```python
from build123d import *

# Parameters (mm, degrees)
SKETCH1_W             = 30
SKETCH1_H             = 18
BOSS_EXTRUDE1_DEPTH   = 30
SKETCH2_R             = 1.25
CUT_EXTRUDE1_DEPTH    = 8
SKETCH3_R             = 4
CUT_EXTRUDE2_DEPTH    = 6.5
SKETCH4_R             = 2.1
CUT_EXTRUDE3_DEPTH    = 24.5
CUT_EXTRUDE4_REACH    = 32
SKETCH5_W             = 12
SKETCH5_H             = 2.5
SKETCH6_R             = 3.45
CUT_EXTRUDE5_DEPTH    = 14
SKETCH7_R             = 1.25
CUT_EXTRUDE6_DEPTH    = 19
CHAMFER1_SIZE         = 1.7
CHAMFER1_SIZE2        = 0.65256886
CHAMFER1_PART_2_SIZE  = 1.7
CHAMFER1_PART_2_SIZE2 = 0.65256886


with BuildPart() as part:
    # Sketch1 → Boss-Extrude1 (new body)
    with BuildSketch(Plane(origin=(0, 0, 0), x_dir=(1, 0, 0), z_dir=(0, 1, 0))):
        Rectangle(SKETCH1_W, SKETCH1_H)
    extrude(amount=BOSS_EXTRUDE1_DEPTH)

    # Sketch2 → Cut-Extrude1 (cut)
    with BuildSketch(Plane(origin=(0, 30, 0), x_dir=(1, 0, 0), z_dir=(0, 1, 0))):
        with Locations((0, -6)):
            Circle(SKETCH2_R)
        with Locations((-8.5, 6)):
            Circle(SKETCH2_R)
        with Locations((8.5, 6)):
            Circle(SKETCH2_R)
    extrude(amount=-CUT_EXTRUDE1_DEPTH, mode=Mode.SUBTRACT)

    # Sketch3 → Cut-Extrude2 (cut)
    with BuildSketch(Plane(origin=(0, 30, 0), x_dir=(1, 0, 0), z_dir=(0, 1, 0))):
        with Locations((-9, -3)):
            Circle(SKETCH3_R)
        with Locations((9, -3)):
            Circle(SKETCH3_R)
    extrude(amount=-CUT_EXTRUDE2_DEPTH, mode=Mode.SUBTRACT)

    # Sketch4 → Cut-Extrude3 (cut, through all)
    with BuildSketch(Plane(origin=(0, 23.5, 0), x_dir=(1, 0, 0), z_dir=(0, 1, 0))):
        with Locations((9, -3)):
            Circle(SKETCH4_R)
        with Locations((-9, -3)):
            Circle(SKETCH4_R)
    extrude(amount=-CUT_EXTRUDE3_DEPTH, mode=Mode.SUBTRACT)

    # Sketch5 → Cut-Extrude4 (cut, up to next)
    with BuildSketch(Plane(origin=(15, 0, 0), x_dir=(0, 0, -1), z_dir=(1, 0, 0)), mode=Mode.PRIVATE) as cut_extrude4_sk1:
        with Locations((9, 7)):
            Rectangle(SKETCH5_W, SKETCH5_H)
    cut_extrude4_tool1 = extrude(cut_extrude4_sk1.sketch, amount=-CUT_EXTRUDE4_REACH, mode=Mode.PRIVATE) & part.part
    add(cut_extrude4_tool1.solids().sort_by_distance((15, 7, -9))[0], mode=Mode.SUBTRACT)
    # Sketch5 → Cut-Extrude4 (cut, up to next)
    with BuildSketch(Plane(origin=(15, 0, 0), x_dir=(0, 0, -1), z_dir=(1, 0, 0)), mode=Mode.PRIVATE) as cut_extrude4_sk2:
        with Locations((9, 11)):
            Rectangle(SKETCH5_W, SKETCH5_H)
    cut_extrude4_tool2 = extrude(cut_extrude4_sk2.sketch, amount=-CUT_EXTRUDE4_REACH, mode=Mode.PRIVATE) & part.part
    add(cut_extrude4_tool2.solids().sort_by_distance((15, 11, -9))[0], mode=Mode.SUBTRACT)
    # Sketch5 → Cut-Extrude4 (cut, up to next)
    with BuildSketch(Plane(origin=(15, 0, 0), x_dir=(0, 0, -1), z_dir=(1, 0, 0)), mode=Mode.PRIVATE) as cut_extrude4_sk3:
        with Locations((9, 15)):
            Rectangle(SKETCH5_W, SKETCH5_H)
    cut_extrude4_tool3 = extrude(cut_extrude4_sk3.sketch, amount=-CUT_EXTRUDE4_REACH, mode=Mode.PRIVATE) & part.part
    add(cut_extrude4_tool3.solids().sort_by_distance((15, 15, -9))[0], mode=Mode.SUBTRACT)
    # Sketch5 → Cut-Extrude4 (cut, up to next)
    with BuildSketch(Plane(origin=(15, 0, 0), x_dir=(0, 0, -1), z_dir=(1, 0, 0)), mode=Mode.PRIVATE) as cut_extrude4_sk4:
        with Locations((9, 19)):
            Rectangle(SKETCH5_W, SKETCH5_H)
    cut_extrude4_tool4 = extrude(cut_extrude4_sk4.sketch, amount=-CUT_EXTRUDE4_REACH, mode=Mode.PRIVATE) & part.part
    add(cut_extrude4_tool4.solids().sort_by_distance((15, 19, -9))[0], mode=Mode.SUBTRACT)
    # Sketch5 → Cut-Extrude4 (cut, up to next)
    with BuildSketch(Plane(origin=(15, 0, 0), x_dir=(0, 0, -1), z_dir=(1, 0, 0)), mode=Mode.PRIVATE) as cut_extrude4_sk5:
        with Locations((9, 23)):
            Rectangle(SKETCH5_W, SKETCH5_H)
    cut_extrude4_tool5 = extrude(cut_extrude4_sk5.sketch, amount=-CUT_EXTRUDE4_REACH, mode=Mode.PRIVATE) & part.part
    add(cut_extrude4_tool5.solids().sort_by_distance((15, 23, -9))[0], mode=Mode.SUBTRACT)
    # Sketch5 → Cut-Extrude4 (cut, up to next)
    with BuildSketch(Plane(origin=(15, 0, 0), x_dir=(0, 0, -1), z_dir=(1, 0, 0)), mode=Mode.PRIVATE) as cut_extrude4_sk6:
        with Locations((9, 27)):
            Rectangle(SKETCH5_W, SKETCH5_H)
    cut_extrude4_tool6 = extrude(cut_extrude4_sk6.sketch, amount=-CUT_EXTRUDE4_REACH, mode=Mode.PRIVATE) & part.part
    add(cut_extrude4_tool6.solids().sort_by_distance((15, 27, -9))[0], mode=Mode.SUBTRACT)
    # Sketch5 → Cut-Extrude4 (cut, up to next)
    with BuildSketch(Plane(origin=(15, 0, 0), x_dir=(0, 0, -1), z_dir=(1, 0, 0)), mode=Mode.PRIVATE) as cut_extrude4_sk7:
        with Locations((9, 3)):
            Rectangle(SKETCH5_W, SKETCH5_H)
    cut_extrude4_tool7 = extrude(cut_extrude4_sk7.sketch, amount=-CUT_EXTRUDE4_REACH, mode=Mode.PRIVATE) & part.part
    add(cut_extrude4_tool7.solids().sort_by_distance((15, 3, -9))[0], mode=Mode.SUBTRACT)

    # Sketch6 → Cut-Extrude5 (cut)
    with BuildSketch(Plane.XZ):
        with Locations((9, 3)):
            Circle(SKETCH6_R)
        with Locations((-9, 3)):
            Circle(SKETCH6_R)
    extrude(amount=-CUT_EXTRUDE5_DEPTH, mode=Mode.SUBTRACT)

    # Sketch7 → Cut-Extrude6 (cut, through all)
    with BuildSketch(Plane.XY.offset(9)):
        with Locations((-4.5, 20)):
            Circle(SKETCH7_R)
        with Locations((4.5, 20)):
            Circle(SKETCH7_R)
        with Locations((-9, 11)):
            Circle(SKETCH7_R)
        with Locations((-9, 3)):
            Circle(SKETCH7_R)
        with Locations((9, 11)):
            Circle(SKETCH7_R)
        with Locations((9, 3)):
            Circle(SKETCH7_R)
        with Locations((0, 10)):
            Circle(SKETCH7_R)
    extrude(amount=-CUT_EXTRUDE6_DEPTH, mode=Mode.SUBTRACT)

    # Chamfer1
    chamfer1_edges = [part.edges().sort_by_distance(p)[0] for p in [
        (6.9, 23.5, 3),
    ]]
    chamfer1_side = [part.faces().sort_by_distance(p)[0] for p in [
        (5.113137085, 23.5, 3),
    ]]
    chamfer(chamfer1_edges, length=CHAMFER1_SIZE, length2=CHAMFER1_SIZE2, reference=chamfer1_side[0])

    # Chamfer1 part 2
    chamfer1_part_2_edges = [part.edges().sort_by_distance(p)[0] for p in [
        (-11.1, 23.5, 3),
    ]]
    chamfer1_part_2_side = [part.faces().sort_by_distance(p)[0] for p in [
        (-12.886862915, 23.5, 3),
    ]]
    chamfer(chamfer1_part_2_edges, length=CHAMFER1_PART_2_SIZE, length2=CHAMFER1_PART_2_SIZE2, reference=chamfer1_part_2_side[0])


solid = part.part
```
The model under review builds one solid part; all positions refer to its coordinate system, in mm. A direction names the side the tool comes from. Round coordinates to 2 decimals unless told otherwise and drop trailing zeros. Answer in a Markdown table with one row per item.
(1) Take a section at C-C on x = 8.5. Count the separate pieces of the cut face and the enclosed holes in it, plus the area to 3 significant figures.
Result set:
| item | result |
|---|---|
| separate pieces | 8 |
| enclosed holes | 0 |
| area | 216 mm2 |
(2) Clearance check with flat-ended pins moving along their axes: P1, Ø3, axis at x = 0, z = 6, coming from the +Y side; P2, Ø5, axis at x = 9, z = 3, coming from the -Y side; P3, Ø0.8, axis at x = 11, y = 3.5, coming from the -Z side. State where each tip first meets the part, or that it passes through.
Result set:
| item | result |
|---|---|
| P1 | stops at y = 30 |
| P2 | stops at y = 14 |
| P3 | stops at z = -3 |
(3) Machinability: for faces 1 (the face through (0, 28.25, -6)), 2 (the face through (-0.27, 26.06, 7.22)), 3 (the face through (0, 5, -9)), which of the approach directions +Z, -Z, +X, -X, +Y, -Y give a long, thin tool a straight path to every point of the face, cutting with its end or side? Answer none if there is none.
Result set:
| item | result |
|---|---|
| face 1 | -Z, +X, -X |
| face 2 | +Y |
| face 3 | -Z, +X, -X, +Y, -Y |
(4) Mouldability with a two-part tool opening along X and no side actions: class faces 4 (the face through (-0.2, 8.5, -9)), 5 (the face through (-15, 15, 2)), 6 (the face through (7.75, 11.05, -1.59)) as released by +X, released by -X, zero draft, split by the parting line, or undercut.
Result set:
| item | result |
|---|---|
| face 4 | zero draft |
| face 5 | released by -X |
| face 6 | undercut |
(5) For line 1 (X direction, y = 28.7, z = -6); line 2 (X direction, y = 3, z = 1); line 3 (Z direction, x = -8.5, y = 25.35), list the stretches that pass through material, from the lowest coordinate up. Write a range as from..to.
Result set:
| item | result |
|---|---|
| line 1 | x = -15..-9.75, -7.25..7.25, 9.75..15 |
| line 2 | x = -15..-11.81, -6.19..6.19, 11.81..15 |
| line 3 | z = -9..-7.25, -4.75..-0.97, 6.97..9 |
